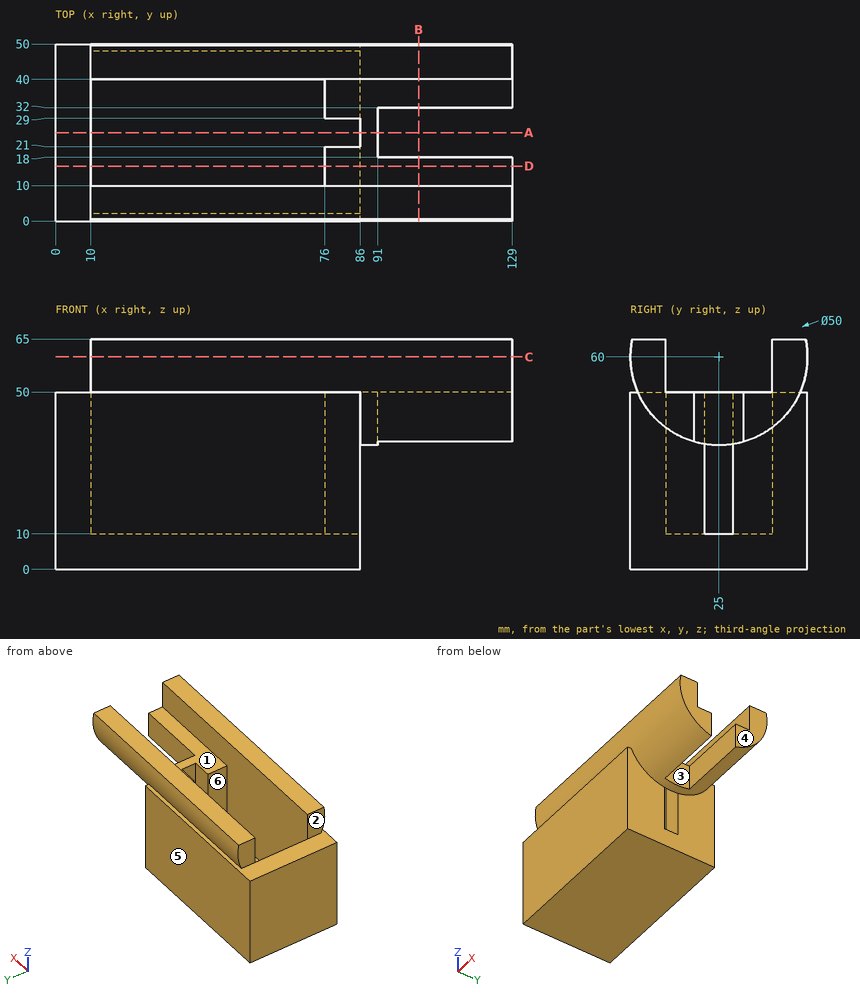
The figure shows three views and two pictorial views of one solid part (mm, origin at its lowest corner). Answer the questions. A direction names the side the tool comes from. Coordinates: 2 decimals unless noted, no trailing zeros. Order: outer loops, then holes, each group sorted by start corner. A loop starts at its lowest first (then second) coordinate and runs counter-clockwise, first axis right, second up.
Q1. A cutting plane is placed at B-B, the plane x = 102.5. Write down the section's boundary in (y, z).
Q2. For a pull along X with two mould halves and no side action, classify the marked faces 4, 5 and 6 as pulls with the +X half, pulls with the -X half, needs draft (parallel to the pull), parting line crosses it, or undercut.
Q3. A cutting plane is placed at A-A, the plane y = 25. Write down the section's boundary in (x, z).
Q4. Which of the six approach directions +Z, -Z, +X, -X, +Y, -Y give full straight-line access (tool end or side, diameter ignored) to the marked faces 1, 2 and 3?
Q5. Consider line 1 (X direction, y = 31, z = 47); line 2 (X direction, y = 34, z = 30.5); line 3 (Y direction, x = 26, z = 61). Determine where each line is inside the solid, lowest interval first.
Q6. A cutting plane is placed at C-C, the plane z = 60. Write down the section's boundary in (x, y), and give its area (3 significant figures).
Q7. Given P1, Ø5, axis at x = 75.5, y = 27, coming from the +Z side; P2, Ø7, axis at x = 119, z = 42.5, coming from the -Y side; P3, Ø8, axis at y = 3, z = 56.5, coming from the -X side, each flat-ended and moving along its own axis, determine where each tip first touches the part or whether it passes through.
Q8. A cutting plane is placed at D-D, the plane y = 15.5. Write down the section's boundary in (x, z), and give its area (3 significant figures).
Answers follow:
1. outline: (0.51, 65) arc R25 ccw to (18, 36) - (18, 50) - (10, 50) - (10, 65) - close; (32, 36) arc R25 ccw to (49.49, 65) - (40, 65) - (40, 50) - (32, 50) - close
2. face 4: pulls with the +X half
2. face 5: needs draft
2. face 6: undercut
3. outline: (0, 0) - (86, 0) - (86, 10) - (10, 10) - (10, 50) - (0, 50) - close; (86, 35) - (91, 35) - (91, 50) - (86, 50) - close
4. face 1: +Z, +X, -X
4. face 2: +Z, -X, +Y, -Y
4. face 3: +Z, -Z, +X
5. line 1: x = 0 to 10, 76 to 91
5. line 2: x = 0 to 10, 76 to 86
5. line 3: y = 0.02 to 10, 40 to 49.98
6. outline: (10, 0) - (129, 0) - (129, 10) - (10, 10) - close; (10, 40) - (129, 40) - (129, 50) - (10, 50) - close
6. area: 2,380 mm2
7. P1: stops at z = 50
7. P2: stops at y = 4.29
7. P3: stops at x = 10
8. outline: (0, 0) - (86, 0) - (86, 36.88) - (129, 36.88) - (129, 50) - (76, 50) - (76, 10) - (10, 10) - (10, 50) - (0, 50) - close
8. area: 2,220 mm2
